```python
from build123d import *

# Parameters (mm, degrees)
SKETCH2_R           = 65
SKETCH2_R_2         = 60
EXTRUDE_THIN1_DEPTH = 50
SKETCH4_W           = 30
SKETCH4_H           = 20
BOSS_EXTRUDE1_DEPTH = 50


with BuildPart() as part:
    # Sketch2 → Extrude-Thin1 (new body)
    with BuildSketch(Plane(origin=(0, 0, 0), x_dir=(1, 0, 0), z_dir=(0, 1, 0))):
        Circle(SKETCH2_R)
        Circle(SKETCH2_R_2, mode=Mode.SUBTRACT)
    extrude(amount=EXTRUDE_THIN1_DEPTH)

    # Sketch3 → Revolve1 (revolve)
    with BuildSketch(Plane(origin=(0, 0, 0), x_dir=(0, 0, -1), z_dir=(1, 0, 0)), mode=Mode.PRIVATE) as revolve1_sk:
        Polygon((-65, 0), (-60, 0), (-37.255621264, -70), (-42.255621264, -70), align=None)
    revolve(revolve1_sk.sketch.rotate(Axis((0, 0, 0), (0, 1, 0)), 180), axis=Axis((0, 0, 0), (0, 1, 0)))

    # Sketch4 → Boss-Extrude1 (add)
    with BuildSketch(Plane(origin=(0, 0, 0), x_dir=(1, 0, 0), z_dir=(0, 1, 0))):
        with Locations((0, -70)):
            Rectangle(SKETCH4_W, SKETCH4_H)
    extrude(amount=BOSS_EXTRUDE1_DEPTH)


solid = part.part
```
For this review, take the finished solid that the model builds, in its own axes (mm). A direction names the side the tool comes from. Coordinates: 2 decimals unless noted, no trailing zeros. Write each loop counter-clockwise with the first axis right and the second up, starting at its lowest first coordinate (ties: lowest second). Pieces come first, ordered by that corner, then holes. Notation, with made-up numbers: (10.5, -16.75) -> (55.5, -16.75) arc R34 cw to (55.5, 17.25) -> close; hole circle Ø4 at (26, 68). An arc over 180 degrees is marked (long way). Put each result on its own line as item: value.
Q1. Take a section at A-A, the plane y = 41.5. State the section outline as (x, z) points, then the cut area to 3 significant figures.
From the geometry:
outline: (-15, 63.25) arc R65 ccw (long way) to (15, 63.25) -> (15, 80) -> (-15, 80) -> close; hole circle Ø120 at (0, 0)
area: 2,430 mm2
Q2. Tool access review of faces 1 (the flat face through (-15, 25, 72)), 2 (the cylindrical face through (-59.94, 24.65, -2.64)), 3 (the flat face through (0, 50, 61)), 4 (the flat face through (15, 25, 72)): name each direction out of +Z, -Z, +X, -X, +Y, -Y from which nothing blocks a thin tool from reaching the whole face with its end or side.
From the geometry:
face 1: +Z, -X, +Y, -Y
face 2: +Y
face 3: +Z, -Z, +X, -X, +Y
face 4: +Z, +X, +Y, -Y
Q3. Take a section at B-B, the plane x = 0. State the section outline as (y, z) points.
From the geometry:
outline: (-70, -42.26) -> (0, -65) -> (50, -65) -> (50, -60) -> (0, -60) -> (-70, -37.26) -> close; (-70, 37.26) -> (0, 60) -> (50, 60) -> (50, 80) -> (0, 80) -> (0, 65) -> (-70, 42.26) -> close
Q4. Take a section at D-D, the plane y = -30. State the section outline as (x, z) points.
From the geometry:
outline: circle Ø110.5 at (0, 0); hole circle Ø100.5 at (0, 0)
Q5. Clearance check with flat-ended pins moving along their axes: pin 1 Ø1.5 at (x, y) = (21, 33) entering from -Z; pin 2 Ø2 at (x, y) = (-4.5, 25) entering from -Z; pin 3 Ø10 at (y, z) = (32.5, 16) entering from -X; pin 4 Ø10 at (x, z) = (-29, 64) entering from -Y. State where each tip first meets the part, or that it passes through.
From the geometry:
pin 1: stops at z = -61.77
pin 2: stops at z = -64.91
pin 3: stops at x = -64.06
pin 4: passes through
Q6. Wall thickness on L1, parallel to Z at x = 0, y = 27; L2, parallel to X at y = 20, z = 0; L3, parallel to Z at x = 18, y = 14: over which ranges is each line inside the solid? List them lowest first.
From the geometry:
L1: z = -65 to -60, 60 to 80
L2: x = -65 to -60, 60 to 65
L3: z = -62.46 to -57.24, 57.24 to 62.46
Q7. Take a section at C-C, the plane z = 0. State the section outline as (x, y) points, then the cut area to 3 significant figures.
From the geometry:
outline: (-65, 0) -> (-42.26, -70) -> (-37.26, -70) -> (-60, 0) -> (-60, 50) -> (-65, 50) -> close; (37.26, -70) -> (42.26, -70) -> (65, 0) -> (65, 50) -> (60, 50) -> (60, 0) -> close
area: 1,200 mm2
